Could you check a few things on this model? Use its own coordinates, in mm. Coordinates: 2 decimals unless noted, no trailing zeros. Loops run counter-clockwise (first coordinate to the right, second up) from the corner with the lowest first, then second, coordinate; pieces in that order, holes last.
1) If I drill on line 1 along Z through (x, y) = (-10.16, 4); line 2 along X through (y, z) = (0.5, -3) (3 decimals); line 3 along X through (y, z) = (4, 0.5) (3 decimals), over which ranges is the centre line in solid material (lowest first)?
2) Thinking about a two-plate mould opening in Z: for faces 1 (the face through (0, 3, -6.35)), 2 (the face through (-4, 0, 0)), 3 (the face through (0.99, 3.22, 3.15)), which applies, released by +Z, released by -Z, zero draft, split by the parting line, or undercut?
3) Imagine slicing it at B-B on y = 2. Please give me the cut outline in (x, z) (3 decimals), plus the area to 3 significant figures.
4) Imagine slicing it at C-C on z = 0. Please give me the cut outline in (x, y) (3 decimals).
5) Imagine slicing it at D-D on z = -2. Please give me the cut outline in (x, y) (3 decimals).
6) Imagine slicing it at A-A on x = 10.16. Please give me the cut outline in (y, z), plus the area to 3 significant figures.
```python
from build123d import *

# Parameters (mm, degrees)
SKETCH1_W             = 31.75
SKETCH1_H             = 12.7
BOSS_EXTRUDE1_DEPTH   = 6.35
CUT_EXTRUDE1_REACH    = 20.239
SKETCH2_R             = 3.302
F_4_CLEARANCE_HOLE1_D = 3.2639


with BuildPart() as part:
    # Sketch1 → Boss-Extrude1 (new body)
    with BuildSketch(Plane(origin=(0, 0, 0), x_dir=(1, 0, 0), z_dir=(0, 1, 0))):
        Rectangle(SKETCH1_W, SKETCH1_H)
    extrude(amount=BOSS_EXTRUDE1_DEPTH)

    # Sketch2 → Cut-Extrude1 (cut, up to next)
    with BuildSketch(Plane(origin=(0, 6.35, 0), x_dir=(1, 0, 0), z_dir=(0, 1, 0)), mode=Mode.PRIVATE) as cut_extrude1_sk1:
        with Locations(Location((0, 0, 0), (0, 0, 270))):
            Circle(SKETCH2_R)
    cut_extrude1_tool1 = extrude(cut_extrude1_sk1.sketch, amount=-CUT_EXTRUDE1_REACH, mode=Mode.PRIVATE) & part.part
    add(cut_extrude1_tool1.solids().sort_by_distance((0, 6.35, 0))[0], mode=Mode.SUBTRACT)

    # #4 Clearance Hole1 (through all)
    with Locations(Plane(origin=(0, 6.35, 0), x_dir=(1, 0, 0), z_dir=(0, 1, 0))):
        with Locations((-10.16, 0)):
            f_4_clearance_hole1 = Hole(F_4_CLEARANCE_HOLE1_D / 2)

    # Mirror1: #4 Clearance Hole1 across plane
    add(f_4_clearance_hole1.mirror(Plane(origin=(0, 0, 0), x_dir=(0, 0, 1), z_dir=(1, 0, 0))), mode=Mode.SUBTRACT)


solid = part.part
```
Filled in:
1. line 1: z = -6.35 to -1.63, 1.63 to 6.35
1. line 2: x = -15.875 to -1.38, 1.38 to 15.875
1. line 3: x = -15.875 to -11.713, -8.607 to -3.264, 3.264 to 8.607, 11.713 to 15.875
2. face 1: released by -Z
2. face 2: zero draft
2. face 3: undercut
3. outline: (-15.875, -6.35) - (15.875, -6.35) - (15.875, 6.35) - (-15.875, 6.35) - close; hole circle Ø3.264 at (-10.16, 0); hole circle Ø6.604 at (0, 0); hole circle Ø3.264 at (10.16, 0)
3. area: 352 mm2
4. outline: (-15.875, 0) - (-11.792, 0) - (-11.792, 6.35) - (-15.875, 6.35) - close; (-8.528, 0) - (-3.302, 0) - (-3.302, 6.35) - (-8.528, 6.35) - close; (3.302, 0) - (8.528, 0) - (8.528, 6.35) - (3.302, 6.35) - close; (11.792, 0) - (15.875, 0) - (15.875, 6.35) - (11.792, 6.35) - close
5. outline: (-15.875, 0) - (-2.627, 0) - (-2.627, 6.35) - (-15.875, 6.35) - close; (2.627, 0) - (15.875, 0) - (15.875, 6.35) - (2.627, 6.35) - close
6. outline: (0, -6.35) - (6.35, -6.35) - (6.35, -1.63) - (0, -1.63) - close; (0, 1.63) - (6.35, 1.63) - (6.35, 6.35) - (0, 6.35) - close
6. area: 59.9 mm2
